```python
from build123d import *

# Parameters (mm, degrees)
EXTRUDE_1_DEPTH     = 115
SKETCH_2_W          = 24.5
SKETCH_2_H          = 27
CUT_EXTRUDE_1_DEPTH = 31


with BuildPart() as part:
    # Эскиз1 → Бобышка-Вытянуть1 (new body)
    with BuildSketch(Plane.XY):
        Polygon((0, 30), (0, 0), (30, 0), (30, 3), (3, 3), (3, 30), align=None)
    extrude(amount=EXTRUDE_1_DEPTH)

    # Эскиз2 → Вырез-Вытянуть1 (cut, through all)
    with BuildSketch(Plane.ZY):
        with Locations((12.25, 16.5)):
            Rectangle(SKETCH_2_W, SKETCH_2_H)
        with Locations((102.75, 16.5)):
            Rectangle(SKETCH_2_W, SKETCH_2_H)
    extrude(amount=-CUT_EXTRUDE_1_DEPTH, mode=Mode.SUBTRACT)


solid = part.part
```
The model under review builds one solid part; all positions refer to its coordinate system, in mm. A direction names the side the tool comes from. Round coordinates to 2 decimals unless told otherwise and drop trailing zeros. Loops run counter-clockwise (first coordinate to the right, second up) from the corner with the lowest first, then second, coordinate; pieces in that order, holes last. Notation, with made-up numbers: (0.25, 43) - (50.25, 43) arc R21 ccw to (50.25, 59) - close; hole circle Ø10 at (-31, 66.25). An arc over 180 degrees is marked (long way). Write each question's results on one line, items separated by ' | '. Start each with the question number.
Q1. Take a section at C-C on y = 18.5. Give the boundary of the cut face in (x, z), plus the area to 3 significant figures.
Q2. Take a section at B-B on x = 17.5. Give the boundary of the cut face in (y, z).
Q3. Tool access review of faces 1 (the flat face through (1, 16, 24.5)), 2 (the flat face through (3, 16, 57)), 3 (the flat face through (1, 16, 90.5)), 4 (the flat face through (30, 1, 57)), 5 (the flat face through (15, 2, 0)): name each direction out of +Z, -Z, +X, -X, +Y, -Y from which nothing blocks a thin tool from reaching the whole face with its end or side.
Q4. Wall thickness on line 1 along Y through (x, z) = (19, 55); line 2 along Z through (x, y) = (2.25, 24.5): over which ranges is each line inside the solid? List them lowest first. Write a range as [from, to].
Q5. Insertion check: P1, Ø5, axis at y = 20.5, z = 88.5, coming from the +X side; P2, Ø12, axis at x = 3.5, z = 65, coming from the +Y side; P3, Ø1, axis at x = 5, y = 13.5, coming from the -Z side; P4, Ø0.9, axis at x = 1, y = 11.5, coming from the -Z side. Each pin has a flat end and moves straight along its axis. Give the tip position at first contact, or say it passes through.
Q6. Take a section at A-A on z = 74.5. Give the boundary of the cut face in (x, y), plus the area to 3 significant figures.
Data:
1) outline: (0, 24.5) - (3, 24.5) - (3, 90.5) - (0, 90.5) - close | area: 198 mm²
2) outline: (0, 0) - (3, 0) - (3, 115) - (0, 115) - close
3) face 1: -Z, +X, -X, +Y | face 2: +Z, -Z, +X, +Y | face 3: +Z, +X, -X, +Y | face 4: +Z, -Z, +X, +Y, -Y | face 5: -Z, +X, -X, +Y, -Y
4) line 1: y = [0, 3] | line 2: z = [24.5, 90.5]
5) P1: stops at x = 3 | P2: stops at y = 30 | P3: passes through | P4: stops at z = 24.5
6) outline: (0, 0) - (30, 0) - (30, 3) - (3, 3) - (3, 30) - (0, 30) - close | area: 171 mm²
